Geometry check sheet. Reference: the model listing, model coordinates, mm. A direction names the side the tool comes from. Coordinates: 2 decimals unless noted, no trailing zeros. Order: outer loops, then holes, each group sorted by start corner. A loop starts at its lowest first (then second) coordinate and runs counter-clockwise, first axis right, second up. Notation, with made-up numbers: (2, 6.25) - (41, 6.25) arc R18 ccw to (41, 31.25) - close; hole circle Ø2 at (73.25, 31.5). An arc over 180 degrees is marked (long way). Use CSV: the item, a comma, the result in double quotes. Start each with the question number.
1) Sectioned sample at B-B, the plane x = 42. Record the cut outline in (y, z).
2) Sectioned sample at D-D, the plane y = -30. Record the cut outline in (x, z).
3) Thickness scan on probe 1 along Y at (x, z) = (67, 5); probe 2 along Z at (x, y) = (3, 0); probe 3 along X at (y, z) = (10.5, -22). Record the ranges inside material, lowest first. Write a range as [from, to].
4) Depth check by flat-ended pin: P1, Ø3, axis at y = 15, z = -18, coming from the +X side; P2, Ø10, axis at x = 9, y = 17, coming from the -Z side; P3, Ø5, axis at x = 27.5, z = 22, coming from the +Y side. Enter the tip coordinate at first touch or a pass-through.
5) Sectioned sample at C-C, the plane z = 0. Record the cut outline in (x, y).
6) Draft check along Y on faces 1 (the flat face through (39, -37, 22.15)), 2 (the flat face through (37, -40, 0)), 3 (the flat face through (2, 28, 28)), 4 (the cylindrical face through (2.46, -18.74, 15.66)). Enter one of: released by +Y, released by -Y, zero draft, split by the parting line, or undercut.
7) Sectioned sample at A-A, the plane y = 0. Record the cut outline in (x, z).
8) Tool access check on faces 5 (the flat face through (37, -35, 0)), 6 (the flat face through (0, -18, 14)), 7 (the flat face through (39, -37, 17.85)). Record the directions out of +Z, -Z, +X, -X, +Y, -Y that give a thin tool (end or side, any length) a straight path to the whole face; none if there is none.
Autodesk Inventor part; units mm, degrees
ref_plane "YZ Plane" through (0, 0, 0) normal (1, 0, 0) x (0, 1, 0)
ref_plane "XZ Plane" through (0, 0, 0) normal (0, 1, 0) x (-1, 0, 0)
ref_plane "XY Plane" through (0, 0, 0) normal (0, 0, 1) x (1, 0, 0)
sketch "Sketch5" plane through (0, 0, 0) normal (1, 0, 0) x (0, 1, 0)
  line L0 (30, 30) -> (30, -30)
  line L1 (30, -30) -> (-35, -30)
  line L2 (-35, -30) -> (-35, 30)
  line L3 (30, 30) -> (-35, 30)
  circle A0 centre (0, 0) radius 20.5
  circle A1 centre (18.385, 18.385) radius 2.75
  circle A2 centre (18.385, -18.385) radius 2.75
  circle A3 centre (-18.385, 18.385) radius 2.75
  circle A4 centre (-18.385, -18.385) radius 2.75
  dimension "d47" = 60
  dimension "d48" = 65
  dimension "d49" = 60
  dimension "d50" = 41
  dimension "d55" = 5.5
  dimension "d56" = 5.5
  dimension "d57" = 5.5
  dimension "d58" = 5.5
extrude "Extrusion5" add sketch "Sketch5" along normal blind 5
sketch "Sketch6" plane through (0, -35, -30) normal (0, -1, 0) x (1, 0, 0)
  line L0 (0, 60) -> (0, 0)
  line L1 (0, 60) -> (70, 60)
  line L2 (70, 60) -> (70, 0)
  line L3 (70, 0) -> (0, 0)
  line L4 (0, 0) -> (0, 60)
  line L5 (70, 60) -> (59.8, 60)
  arc A0 (59.8, 47.85) -> (59.8, 52.15) centre (59.8, 50) ccw
  arc A1 (59.8, 7.85) -> (59.8, 12.15) centre (59.8, 10) ccw
  arc A2 (18.1, 52.15) -> (18.1, 47.85) centre (18.1, 50) ccw
  arc A3 (18.1, 12.15) -> (18.1, 7.85) centre (18.1, 10) ccw
  line L6 (59.8, 47.85) -> (18.1, 47.85)
  line L7 (59.8, 52.15) -> (18.1, 52.15)
  line L8 (59.8, 7.85) -> (18.1, 7.85)
  line L9 (59.8, 12.15) -> (18.1, 12.15)
  point P0 (0, 30)
  dimension "d61" = 70
  dimension "d62" = 60
  dimension "d65" = 4.3
  dimension "d67" = 4.3
  dimension "d69" = 4.3
  dimension "d71" = 4.3
extrude "Extrusion6" add sketch "Sketch6" along normal blind 5
chamfer "Chamfer1" distance 4 angle 45 1 edges at (2.5, 30, -30)
chamfer "Chamfer2" distance 4 angle 45 1 edges at (2.5, 30, 30)
chamfer "Chamfer3" distance 4 angle 45 1 edges at (70, -37.5, 30)
chamfer "Chamfer4" distance 4 angle 45 1 edges at (70, -37.5, -30)
fillet "Fillet2" radius 4 1 edges at (0, -40, 0)
sketch "Sketch7" plane through (0, 26, 30) normal (0, 0, 1) x (1, 0, 0)
  line L0 (5, -61) -> (66, -61)
  line L1 (5, -61) -> (25, -61)
  line L2 (5, -61) -> (5, -41)
  line L3 (5, -61) -> (5, 0)
  line L4 (5, -41) -> (25, -61)
  point P0 (0, -26)
  dimension "d87" = 20
  dimension "d88" = 20
extrude "Extrusion7" add sketch "Sketch7" against normal blind 3
sketch "Sketch8" plane through (5, 26, -30) normal (0, 0, -1) x (-1, 0, 0)
  line L0 (0, -61) -> (-61, -61)
  line L1 (0, 0) -> (0, -41)
  line L2 (0, -61) -> (0, -41)
  line L3 (-20, -61) -> (0, -41)
  line L4 (0, -61) -> (-20, -61)
  line L5 (-20, -61) -> (0, -41)
  point P0 (5, -26)
extrude "Extrusion8" add sketch "Sketch8" against normal blind 3
properties part number "mount" material "Aluminum 6061"
Evaluation:
1,outline,"(-40, -30) - (-35, -30) - (-35, -22.15) - (-40, -22.15) - close; (-40, -17.85) - (-35, -17.85) - (-35, 17.85) - (-40, 17.85) - close; (-40, 22.15) - (-35, 22.15) - (-35, 30) - (-40, 30) - close"
2,outline,"(0, -30) - (20, -30) - (20, -27) - (5, -27) - (5, 27) - (20, 27) - (20, 30) - (0, 30) - close"
3,probe 1,"[-40, -35]"
3,probe 2,"[-30, -20.5], [20.5, 30]"
3,probe 3,"[0, 5]"
4,P1,"x = 5"
4,P2,"z = -30"
4,P3,"y = -35"
5,outline,"(0, -36) arc R4 ccw to (4, -40) - (70, -40) - (70, -35) - (5, -35) - (5, -20.5) - (0, -20.5) - close; (0, 20.5) - (5, 20.5) - (5, 30) - (0, 30) - close"
6,face 1,"zero draft"
6,face 2,"released by -Y"
6,face 3,"released by +Y"
6,face 4,"undercut"
7,outline,"(0, -30) - (5, -30) - (5, -20.5) - (0, -20.5) - close; (0, 20.5) - (5, 20.5) - (5, 30) - (0, 30) - close"
8,face 5,"+X, +Y"
8,face 6,"+Z, -Z, -X, +Y, -Y"
8,face 7,"+Y, -Y"
